Here's how the part is built. I have some questions about the finished solid (model axes, mm). A direction names the side the tool comes from. Round coordinates to 2 decimals unless told otherwise and drop trailing zeros. Use a Markdown table: item, result.
```python
from build123d import *

# Parameters (mm, degrees)
F0_W     = 50.8
F0_H     = 19.05
F1_DEPTH = 774.7
F2_W     = 122.43557321
F2_H     = 50.8
F2_W_2   = 343.1604206562
F3_DEPTH = 25.4
F4_R     = 0.79375
F5_DEPTH = 25.4
F6_R     = 4.7625
F7_DEPTH = 25.4


# Not quite as in the source:
# - a feature names something its author has since deleted; it is built from what else it names


with BuildPart() as f1:
    # F0 (on Top) → F1 (new body)
    with BuildSketch(Plane.XY):
        Rectangle(F0_W, F0_H)
    extrude(amount=F1_DEPTH)

    # F2 (on Front) → F3 (cut)
    with BuildSketch(Plane.XZ):
        with Locations((22.4465244144, 25.4)):
            Rectangle(F2_W, F2_H)
        with Locations((-38.7818217278, 749.3)):
            Rectangle(F2_W_2, F2_H)
    extrude(amount=F3_DEPTH, mode=Mode.SUBTRACT)

    # F4 (on Front) → F5 (cut)
    with BuildSketch(Plane.XZ):
        with Locations((9.525, 101.6)):
            Circle(F4_R)
        with Locations((9.525, 155.575)):
            Circle(F4_R)
        with Locations((9.525, 619.125)):
            Circle(F4_R)
        with Locations((9.525, 673.1)):
            Circle(F4_R)
        with Locations((-9.525, 619.125)):
            Circle(F4_R)
        with Locations((-9.525, 673.1)):
            Circle(F4_R)
        with Locations((-9.525, 101.6)):
            Circle(F4_R)
        with Locations((-9.525, 155.575)):
            Circle(F4_R)
    extrude(amount=-F5_DEPTH, mode=Mode.SUBTRACT)

    # F6 (on Front) → F7 (cut)
    with BuildSketch(Plane.XZ):
        with Locations((0, 95.25)):
            Circle(F6_R)
        with Locations((0, 361.95)):
            Circle(F6_R)
    extrude(amount=F7_DEPTH, mode=Mode.SUBTRACT)


solid = f1.part
```
Q1. Will these pins go through, and if not, where does the flat tip stop? P1, Ø4, axis at x = -7.5, y = -2.5, coming from the +Z side; P2, Ø3, axis at x = -0.5, z = 361, coming from the -Y side; P3, Ø3, axis at x = -1.5, y = -5.5, coming from the -Z side.
Return value:
| item | result |
|---|---|
| P1 | stops at z = 723.9 |
| P2 | stops at y = 0 |
| P3 | stops at z = 50.8 |
Q2. I need wall thicknesses on line 1 (Z direction, x = 0, y = -6.5); line 2 (Z direction, x = -1, y = -3.25); line 3 (X direction, y = -2.5, z = 95.25). Which ranges of each line are inside material? Lowest first, please. Write a range as from..to.
Return value:
| item | result |
|---|---|
| line 1 | z = 50.8..90.49, 100.01..357.19, 366.71..723.9 |
| line 2 | z = 50.8..90.59, 99.91..357.29, 366.61..723.9 |
| line 3 | x = -25.4..-4.76, 4.76..25.4 |
Q3. For faces 1 (the flat face through (0, 0, 750)), 2 (the flat face through (0, 0, 26)), 3 (the flat face through (-25.4, 0, 382)), which set-ups out of +Z, -Z, +X, -X, +Y, -Y let a thin tool reach every point of the face, with its end or its side?
Return value:
| item | result |
|---|---|
| face 1 | +Z, +X, -X, -Y |
| face 2 | -Z, +X, -X, -Y |
| face 3 | +Z, -Z, -X, +Y, -Y |
Q4. Imagine slicing it at A-A, the plane y = -5.5. Give the number of separate pieces and of enclosed holes in the cut face, then the cut area to 3 significant figures.
Return value:
| item | result |
|---|---|
| separate pieces | 1 |
| enclosed holes | 2 |
| area | 34,100 mm^2 |
